from build123d import *

# Parameters (mm, degrees)
SKETCH1_W           = 45
SKETCH1_H           = 25
BOSS_EXTRUDE1_DEPTH = 1
SKETCH2_R           = 1.5
CUT_EXTRUDE1_DEPTH  = 2
FILLET1_R           = 1


with BuildPart() as part:
    # Sketch1 → Boss-Extrude1 (new body)
    with BuildSketch(Plane.XY):
        Rectangle(SKETCH1_W, SKETCH1_H)
    extrude(amount=BOSS_EXTRUDE1_DEPTH)

    # Sketch2 → Cut-Extrude1 (cut, through all)
    with BuildSketch(Plane.XY.offset(1)):
        with Locations((17, 7.5)):
            Circle(SKETCH2_R)
        with Locations((10, 7.5)):
            Circle(SKETCH2_R)
        with Locations((-17, 7.5)):
            Circle(SKETCH2_R)
        with Locations((-10, 7.5)):
            Circle(SKETCH2_R)
        with Locations((17, -7.5)):
            Circle(SKETCH2_R)
        with Locations((10, -7.5)):
            Circle(SKETCH2_R)
        with Locations((-17, -7.5)):
            Circle(SKETCH2_R)
        with Locations((-10, -7.5)):
            Circle(SKETCH2_R)
    extrude(amount=-CUT_EXTRUDE1_DEPTH, mode=Mode.SUBTRACT)

    # Fillet1
    fillet1_edges = [part.edges().sort_by_distance(p)[0] for p in [
        (22.5, -12.5, 0.5),
        (-22.5, -12.5, 0.5),
        (-22.5, 12.5, 0.5),
        (22.5, 12.5, 0.5),
    ]]
    fillet(fillet1_edges, radius=FILLET1_R)


solid = part.part
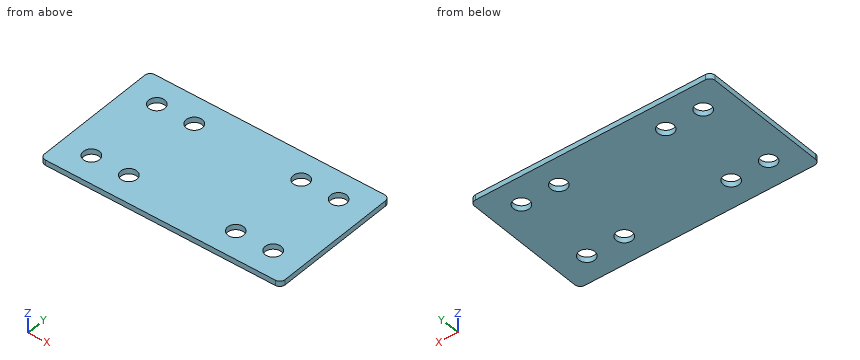
Can you work these out from the model? Positions are in its coordinate system, mm. Round coordinates to 2 decimals unless told otherwise and drop trailing zeros. Order: outer loops, then holes, each group sorted by start corner. A loop starts at its lowest first (then second) coordinate and runs counter-clockwise, first axis right, second up. Notation, with made-up numbers: (-10.5, -23.75) - (36.5, -23.75) arc R27 ccw to (36.5, -3.75) - close; hole circle Ø4 at (32.5, 41). An arc over 180 degrees is marked (long way). Answer in a Markdown table with one row per item.
(1) For P1, Ø8, axis at x = -3, y = 1.5, coming from the -Z side; P2, Ø2.5, axis at x = -17, y = 7.5, coming from the -Z side, each with a flat end and sliding along its axis, tell me the tip position at first contact or that it passes through.
From the geometry:
| item | result |
|---|---|
| P1 | stops at z = 0 |
| P2 | passes through |
(2) Suppose I cut it at C-C, the plane x = 17. Please give me the cut outline in (y, z).
From the geometry:
| item | result |
|---|---|
| outline | (-12.5, 0) - (-9, 0) - (-9, 1) - (-12.5, 1) - close; (-6, 0) - (6, 0) - (6, 1) - (-6, 1) - close; (9, 0) - (12.5, 0) - (12.5, 1) - (9, 1) - close |
(3) Suppose I cut it at A-A, the plane y = -7.5. Please give me the cut outline in (x, z).
From the geometry:
| item | result |
|---|---|
| outline | (-22.5, 0) - (-18.5, 0) - (-18.5, 1) - (-22.5, 1) - close; (-15.5, 0) - (-11.5, 0) - (-11.5, 1) - (-15.5, 1) - close; (-8.5, 0) - (8.5, 0) - (8.5, 1) - (-8.5, 1) - close; (11.5, 0) - (15.5, 0) - (15.5, 1) - (11.5, 1) - close; (18.5, 0) - (22.5, 0) - (22.5, 1) - (18.5, 1) - close |
(4) Please list where these lines run through material, in increasing order: L1, parallel to Y at x = 17, z = 0.6; L2, parallel to Y at x = -9, z = 0.5; L3, parallel to X at y = -8.75, z = 0.95. Write a range as from..to.
From the geometry:
| item | result |
|---|---|
| L1 | y = -12.5..-9, -6..6, 9..12.5 |
| L2 | y = -12.5..-8.62, -6.38..6.38, 8.62..12.5 |
| L3 | x = -22.5..-17.83, -16.17..-10.83, -9.17..9.17, 10.83..16.17, 17.83..22.5 |
(5) Suppose I cut it at B-B, the plane z = 0.7. Count the separate pieces of the cut face and the enclosed holes in it, plus the area to 3 significant figures.
From the geometry:
| item | result |
|---|---|
| separate pieces | 1 |
| enclosed holes | 8 |
| area | 1,070 mm2 |
